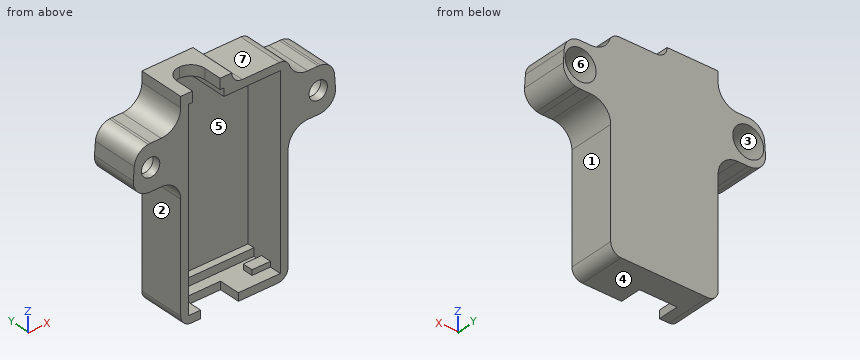
from build123d import *

# Parameters (mm, degrees)
SKETCH1_W           = 20.5
SKETCH1_H           = 38.5
SKETCH1_R           = 4.25
SKETCH1_R_2         = 1.75
BOSS_EXTRUDE1_DEPTH = 1.5
SKETCH2_W           = 20.5
SKETCH2_H           = 38.5
BOSS_EXTRUDE2_DEPTH = 7.35
SKETCH3_W           = 17.5
SKETCH3_H           = 35.5
SKETCH3_W_2         = 6.75
SKETCH3_H_2         = 1.5
CUT_EXTRUDE1_DEPTH  = 7.35
SKETCH4_W           = 7.2
SKETCH4_H           = 1.5
CUT_EXTRUDE2_DEPTH  = 4.05
SKETCH6_W           = 17.5
SKETCH6_H           = 1.5
BOSS_EXTRUDE3_DEPTH = 1.35
SKETCH7_W           = 3.5
SKETCH7_H           = 2
BOSS_EXTRUDE4_DEPTH = 1
SKETCH8_R           = 2.95
BOSS_EXTRUDE5_DEPTH = 7.35
FILLET2_R           = 3.75
CUT_EXTRUDE4_START  = -8.85
CUT_EXTRUDE4_DEPTH  = 8.85
FILLET5_R           = 3
SKETCH10_W          = 9.75
SKETCH10_H          = 2
BOSS_EXTRUDE6_DEPTH = 8.85
CUT_EXTRUDE5_REACH  = 47.729
FILLET4_R           = 2


with BuildPart() as part:
    # Sketch1 → Boss-Extrude1 (new body)
    # profile 1 of 5: a face of its own
    with BuildSketch(Plane(origin=(0, 0, 0), x_dir=(1, 0, 0), z_dir=(0, 1, 0))):
        with Locations((0, 11.25)):
            Rectangle(SKETCH1_W, SKETCH1_H)
    # profile 2 of 5: a face of its own
    with BuildSketch(Plane(origin=(0, 0, 0), x_dir=(1, 0, 0), z_dir=(0, 1, 0))):
        with BuildLine():
            Line((-10.25, -4.25), (-10.25, 4.25))
            Line((-10.25, 4.25), (-16, 4.25))
            ThreePointArc((-16, 4.25), (-12.99479618, 3.00520382), (-11.75, 0))
            ThreePointArc((-11.75, 0), (-12.99479618, -3.00520382), (-16, -4.25))
            Line((-16, -4.25), (-10.25, -4.25))
        make_face()
    # profile 3 of 5: a face of its own
    with BuildSketch(Plane(origin=(0, 0, 0), x_dir=(1, 0, 0), z_dir=(0, 1, 0))):
        with Locations((-16, 0)):
            Circle(SKETCH1_R)
        with Locations(Location((-16, 0, 0), (0, 0, 270))):
            Circle(SKETCH1_R_2, mode=Mode.SUBTRACT)
    # profile 4 of 5: a face of its own
    with BuildSketch(Plane(origin=(0, 0, 0), x_dir=(1, 0, 0), z_dir=(0, 1, 0))):
        with BuildLine():
            Line((16, 4.25), (10.25, 4.25))
            Line((10.25, 4.25), (10.25, -4.25))
            Line((10.25, -4.25), (16, -4.25))
            ThreePointArc((16, -4.25), (11.75, 0), (16, 4.25))
        make_face()
    # profile 5 of 5: a face of its own
    with BuildSketch(Plane(origin=(0, 0, 0), x_dir=(1, 0, 0), z_dir=(0, 1, 0))):
        with Locations((16, 0)):
            Circle(SKETCH1_R)
        with Locations(Location((16, 0, 0), (0, 0, 270))):
            Circle(SKETCH1_R_2, mode=Mode.SUBTRACT)
    extrude(amount=BOSS_EXTRUDE1_DEPTH)

    # Sketch2 → Boss-Extrude2 (add)
    with BuildSketch(Plane(origin=(0, 1.5, 0), x_dir=(1, 0, 0), z_dir=(0, 1, 0))):
        with Locations((0, 11.25)):
            Rectangle(SKETCH2_W, SKETCH2_H)
    extrude(amount=BOSS_EXTRUDE2_DEPTH)

    # Sketch3 → Cut-Extrude1 (cut)
    with BuildSketch(Plane.XZ):
        with Locations((0, -11.25)):
            Rectangle(SKETCH3_W, SKETCH3_H)
        with Locations((-5.375, 7.25)):
            Rectangle(SKETCH3_W_2, SKETCH3_H_2)
    extrude(amount=-CUT_EXTRUDE1_DEPTH, mode=Mode.SUBTRACT)

    # Sketch4 → Cut-Extrude2 (cut)
    with BuildSketch(Plane.XZ):
        with Locations((-2.85, -29.75)):
            Rectangle(SKETCH4_W, SKETCH4_H)
    extrude(amount=-CUT_EXTRUDE2_DEPTH, mode=Mode.SUBTRACT)

    # Sketch6 → Boss-Extrude3 (add)
    with BuildSketch(Plane.XZ.offset(-7.35)):
        with Locations((0, -28.25)):
            Rectangle(SKETCH6_W, SKETCH6_H)
    extrude(amount=BOSS_EXTRUDE3_DEPTH)

    # Sketch7 → Boss-Extrude4 (add)
    with BuildSketch(Plane.XY.offset(-29)):
        with Locations((7, 3.25)):
            Rectangle(SKETCH7_W, SKETCH7_H)
    extrude(amount=BOSS_EXTRUDE4_DEPTH)

    # Sketch8 → Boss-Extrude5 (add)
    # profile 1 of 2: a face of its own
    with BuildSketch(Plane(origin=(0, 1.5, 0), x_dir=(1, 0, 0), z_dir=(0, 1, 0))):
        with BuildLine():
            Line((-10.25, -4.25), (-10.25, 4.25))
            Line((-10.25, 4.25), (-16, 4.25))
            ThreePointArc((-16, 4.25), (-20.25, 0), (-16, -4.25))
            Line((-16, -4.25), (-10.25, -4.25))
        make_face()
        with Locations(Location((-16, 0, 0), (0, 0, 270))):
            Circle(SKETCH8_R, mode=Mode.SUBTRACT)
    # profile 2 of 2: a face of its own
    with BuildSketch(Plane(origin=(0, 1.5, 0), x_dir=(1, 0, 0), z_dir=(0, 1, 0))):
        with BuildLine():
            Line((10.25, 4.25), (10.25, -4.25))
            Line((10.25, -4.25), (16, -4.25))
            ThreePointArc((16, -4.25), (20.25, 0), (16, 4.25))
            Line((16, 4.25), (10.25, 4.25))
        make_face()
        with Locations(Location((16, 0, 0), (0, 0, 270))):
            Circle(SKETCH8_R, mode=Mode.SUBTRACT)
    extrude(amount=BOSS_EXTRUDE5_DEPTH)

    # Fillet2
    fillet2_edges = [part.edges().sort_by_distance(p)[0] for p in [
        (10.25, 4.425, -4.25),
        (10.25, 4.425, 4.25),
        (-10.25, 4.425, 4.25),
        (-10.25, 4.425, -4.25),
    ]]
    fillet(fillet2_edges, radius=FILLET2_R - 0.0001)  # a hair under: the kernel refuses the full size

    # Sketch9 → Cut-Extrude4 (cut)
    with BuildSketch(Plane(origin=(0, 8.85, 0), x_dir=(1, 0, 0), z_dir=(0, 1, 0)).offset(CUT_EXTRUDE4_START)):
        with BuildLine():
            Line((-24.982948352, 53.686308531), (-20.952771504, -3.947905519))
            ThreePointArc((-20.952771504, -3.947905519), (-19.171836931, -8.143524448), (-15.185360396, -10.353264474))
            Line((-15.185360396, -10.353264474), (-1.215537244, -12.816521212))
            ThreePointArc((-1.215537244, -12.816521212), (0, -12.922866941), (1.215537244, -12.816521212))
            Line((1.215537244, -12.816521212), (15.185360396, -10.353264474))
            ThreePointArc((15.185360396, -10.353264474), (19.171836931, -8.143524448), (20.952771504, -3.947905519))
            Line((20.952771504, -3.947905519), (24.982948352, 53.686308531))
            ThreePointArc((24.982948352, 53.686308531), (24.995735789, 53.930307371), (25, 54.174603847))
            Line((25, 54.174603847), (25, 107.825396153))
            ThreePointArc((25, 107.825396153), (24.995735789, 108.069692629), (24.982948352, 108.313691469))
            Line((24.982948352, 108.313691469), (20.952771504, 165.947905519))
            ThreePointArc((20.952771504, 165.947905519), (19.171836931, 170.143524448), (15.185360396, 172.353264474))
            Line((15.185360396, 172.353264474), (1.215537244, 174.816521212))
            ThreePointArc((1.215537244, 174.816521212), (0, 174.922866941), (-1.215537244, 174.816521212))
            Line((-1.215537244, 174.816521212), (-15.185360396, 172.353264474))
            ThreePointArc((-15.185360396, 172.353264474), (-19.171836931, 170.143524448), (-20.952771504, 165.947905519))
            Line((-20.952771504, 165.947905519), (-24.982948352, 108.313691469))
            ThreePointArc((-24.982948352, 108.313691469), (-24.995735789, 108.069692629), (-25, 107.825396153))
            Line((-25, 107.825396153), (-25, 54.174603847))
            ThreePointArc((-25, 54.174603847), (-24.995735789, 53.930307371), (-24.982948352, 53.686308531))
        make_face()
        with BuildLine():
            Line((-18.957643404, 165.808392572), (-22.987820251, 108.174178521))
            ThreePointArc((-22.987820251, 108.174178521), (-22.996954135, 107.999893636), (-23, 107.825396153))
            Line((-23, 107.825396153), (-23, 54.174603847))
            ThreePointArc((-23, 54.174603847), (-22.996954135, 54.000106364), (-22.987820251, 53.825821479))
            Line((-22.987820251, 53.825821479), (-18.957643404, -3.808392572))
            ThreePointArc((-18.957643404, -3.808392572), (-17.68554728, -6.805263235), (-14.838064041, -8.383648968))
            Line((-14.838064041, -8.383648968), (-0.868240888, -10.846905706))
            ThreePointArc((-0.868240888, -10.846905706), (0, -10.922866941), (0.868240888, -10.846905706))
            Line((0.868240888, -10.846905706), (14.838064041, -8.383648968))
            ThreePointArc((14.838064041, -8.383648968), (17.68554728, -6.805263235), (18.957643404, -3.808392572))
            Line((18.957643404, -3.808392572), (22.987820251, 53.825821479))
            ThreePointArc((22.987820251, 53.825821479), (22.996954135, 54.000106364), (23, 54.174603847))
            Line((23, 54.174603847), (23, 107.825396153))
            ThreePointArc((23, 107.825396153), (22.996954135, 107.999893636), (22.987820251, 108.174178521))
            Line((22.987820251, 108.174178521), (18.957643404, 165.808392572))
            ThreePointArc((18.957643404, 165.808392572), (17.68554728, 168.805263235), (14.838064041, 170.383648968))
            Line((14.838064041, 170.383648968), (0.868240888, 172.846905706))
            ThreePointArc((0.868240888, 172.846905706), (0, 172.922866941), (-0.868240888, 172.846905706))
            Line((-0.868240888, 172.846905706), (-14.838064041, 170.383648968))
            ThreePointArc((-14.838064041, 170.383648968), (-17.68554728, 168.805263235), (-18.957643404, 165.808392572))
        make_face(mode=Mode.SUBTRACT)
    extrude(amount=CUT_EXTRUDE4_DEPTH, mode=Mode.SUBTRACT)

    # Fillet5
    fillet5_edges = [part.edges().sort_by_distance(p)[0] for p in [
        (-19.402072162, 4.425, -2.547234776),
        (-19.014456867, 4.425, 2.995922195),
        (19.014456867, 4.425, 2.995922195),
        (19.402072162, 4.425, -2.547234776),
    ]]
    fillet(fillet5_edges, radius=FILLET5_R)

    # Sketch10 → Boss-Extrude6 (add)
    with BuildSketch(Plane(origin=(0, 0, 0), x_dir=(1, 0, 0), z_dir=(0, 1, 0))):
        with Locations((-5.375, -9)):
            Rectangle(SKETCH10_W, SKETCH10_H)
    extrude(amount=BOSS_EXTRUDE6_DEPTH)

    # Sketch11 → Cut-Extrude5 (cut, up to next)
    with BuildSketch(Plane.XY.offset(10), mode=Mode.PRIVATE) as cut_extrude5_sk1:
        with BuildLine():
            ThreePointArc((-2.725, 3.5), (-3.50116703, 5.37383297), (-5.375, 6.15))
            Line((-5.375, 6.15), (-5.375, 0.85))
            ThreePointArc((-5.375, 0.85), (-3.50116703, 1.62616703), (-2.725, 3.5))
        make_face()
    cut_extrude5_tool1 = extrude(cut_extrude5_sk1.sketch, amount=-CUT_EXTRUDE5_REACH, mode=Mode.PRIVATE) & part.part
    # Sketch11 → Cut-Extrude5 (cut, up to next)
    with BuildSketch(Plane.XY.offset(10), mode=Mode.PRIVATE) as cut_extrude5_sk2:
        with BuildLine():
            Line((-5.375, 0.85), (-5.375, 6.15))
            ThreePointArc((-5.375, 6.15), (-7.24883297, 5.37383297), (-8.025, 3.5))
            ThreePointArc((-8.025, 3.5), (-7.24883297, 1.62616703), (-5.375, 0.85))
        make_face()
    cut_extrude5_tool2 = extrude(cut_extrude5_sk2.sketch, amount=-CUT_EXTRUDE5_REACH, mode=Mode.PRIVATE) & part.part
    # Sketch11 → Cut-Extrude5 (cut, up to next)
    with BuildSketch(Plane.XY.offset(10), mode=Mode.PRIVATE) as cut_extrude5_sk3:
        with BuildLine():
            ThreePointArc((-2.725, 3.5), (-3.50116703, 5.37383297), (-5.375, 6.15))
            Line((-5.375, 6.15), (-5.375, 0.85))
            ThreePointArc((-5.375, 0.85), (-3.50116703, 1.62616703), (-2.725, 3.5))
        make_face()
    cut_extrude5_tool3 = extrude(cut_extrude5_sk3.sketch, amount=-CUT_EXTRUDE5_REACH, mode=Mode.PRIVATE) & part.part
    # Sketch11 → Cut-Extrude5 (cut, up to next)
    with BuildSketch(Plane.XY.offset(10), mode=Mode.PRIVATE) as cut_extrude5_sk4:
        with BuildLine():
            Line((-5.375, 0.85), (-5.375, 6.15))
            ThreePointArc((-5.375, 6.15), (-7.24883297, 5.37383297), (-8.025, 3.5))
            ThreePointArc((-8.025, 3.5), (-7.24883297, 1.62616703), (-5.375, 0.85))
        make_face()
    cut_extrude5_tool4 = extrude(cut_extrude5_sk4.sketch, amount=-CUT_EXTRUDE5_REACH, mode=Mode.PRIVATE) & part.part
    # Sketch11 → Cut-Extrude5 (cut, up to next)
    with BuildSketch(Plane.XY.offset(10), mode=Mode.PRIVATE) as cut_extrude5_sk5:
        with BuildLine():
            Line((-5.375, 0), (-5.375, 0.85))
            ThreePointArc((-5.375, 0.85), (-7.24883297, 1.62616703), (-8.025, 3.5))
            Line((-8.025, 3.5), (-8.025, 0))
            Line((-8.025, 0), (-5.375, 0))
        make_face()
    cut_extrude5_tool5 = extrude(cut_extrude5_sk5.sketch, amount=-CUT_EXTRUDE5_REACH, mode=Mode.PRIVATE) & part.part
    # Sketch11 → Cut-Extrude5 (cut, up to next)
    with BuildSketch(Plane.XY.offset(10), mode=Mode.PRIVATE) as cut_extrude5_sk6:
        with BuildLine():
            ThreePointArc((-2.725, 3.5), (-3.50116703, 1.62616703), (-5.375, 0.85))
            Line((-5.375, 0.85), (-5.375, 0))
            Line((-5.375, 0), (-2.725, 0))
            Line((-2.725, 0), (-2.725, 3.5))
        make_face()
    cut_extrude5_tool6 = extrude(cut_extrude5_sk6.sketch, amount=-CUT_EXTRUDE5_REACH, mode=Mode.PRIVATE) & part.part
    add(cut_extrude5_tool1.solids().sort_by_distance((-4.250305, 3.5, 10))[0], mode=Mode.SUBTRACT)
    add(cut_extrude5_tool2.solids().sort_by_distance((-6.499695, 3.5, 10))[0], mode=Mode.SUBTRACT)
    add(cut_extrude5_tool3.solids().sort_by_distance((-4.250305, 3.5, 10))[0], mode=Mode.SUBTRACT)
    add(cut_extrude5_tool4.solids().sort_by_distance((-6.499695, 3.5, 10))[0], mode=Mode.SUBTRACT)
    add(cut_extrude5_tool5.solids().sort_by_distance((-6.993859, 0.832642, 10))[0], mode=Mode.SUBTRACT)
    add(cut_extrude5_tool6.solids().sort_by_distance((-3.756141, 0.832642, 10))[0], mode=Mode.SUBTRACT)

    # Fillet4
    fillet4_edges = [part.edges().sort_by_distance(p)[0] for p in [
        (10.25, 4.425, 8),
        (10.25, 4.425, -30.5),
        (-10.25, 4.425, -30.5),
        (-0.5, 4.425, 8),
    ]]
    fillet(fillet4_edges, radius=FILLET4_R - 0.0001)  # a hair under: the kernel refuses the full size


solid = part.part
Design review of the part built by this model. Coordinates are the model's own, in mm. Face numbers are marked on the shaded views. A direction names the side the tool comes from. Give positions to 0.01 mm unless a question says otherwise; leave off trailing zeros. Loops run counter-clockwise (first coordinate to the right, second up) from the corner with the lowest first, then second, coordinate; pieces in that order, holes last. Notation, with made-up numbers: M -23,79 L 15,79 A15 ccw 15,87 Z; hole C -3,27 d6. An arc over 180 degrees is marked long. Write item = value, one per line.
Q1. For the marked faces 1, 2 and 3, list the 3-axis set-ups (+Z, -Z, +X, -X, +Y, -Y) from which the entire face can be reached by the end or side of a thin tool; tool diameter is ignored.
Output values:
face_1 = -Z, +X, +Y, -Y
face_2 = -Z, -X, +Y, -Y
face_3 = +Y
Q2. To check wall thickness, follow line 1 (X direction, y = 2.5, z = -8); line 2 (X direction, y = 3.5, z = -1); line 3 (Z direction, x = 2.5, y = 3.5). State the ranges of each line that lie inside material, in increasing order. Write a range as [from, to].
Output values:
line_1 = [-10.25, -8.75], [8.75, 10.25]
line_2 = [-19.29, -18.78], [-13.22, -8.75], [8.75, 13.22], [18.78, 19.29]
line_3 = [-30.5, -29], [6.5, 8]
Q3. We need section A-A (z = -21). Give the boundary of the cut face in (x, y), plus the area to 3 significant figures.
Output values:
outline = M -10.25,0 L -8.75,0 L -8.75,7.35 L 8.75,7.35 L 8.75,0 L 10.25,0 L 10.25,8.85 L -10.25,8.85 Z
area = 52.8 mm^2
Q4. We need section D-D (x = -11). Give the boundary of the cut face in (y, z).
Output values:
outline = M 0,-5.75 L 8.85,-5.75 L 8.85,5.75 L 0,5.75 Z
Q5. We need section C-C (z = 0). Give the boundary of the cut face in (x, y), plus the area to 3 significant figures.
Output values:
outline = M -19.22,0 L -17.75,0 L -17.75,1.5 L -18.95,1.5 L -18.95,8.85 L -19.22,8.85 Z; M -14.25,0 L -8.75,0 L -8.75,7.35 L 8.75,7.35 L 8.75,0 L 14.25,0 L 14.25,1.5 L 13.05,1.5 L 13.05,8.85 L -13.05,8.85 L -13.05,1.5 L -14.25,1.5 Z; M 17.75,0 L 19.22,0 L 19.22,8.85 L 18.95,8.85 L 18.95,1.5 L 17.75,1.5 Z
area = 114 mm^2
Q6. Draft analysis for pull direction Z (two halves, no side actions). For the marked faces 4, 5, 6 and 7, state which applies: +Z half, -Z half, draft (parallel to the pull), parting line (faces both ways), or undercut.
Output values:
face_4 = -Z half
face_5 = undercut
face_6 = undercut
face_7 = +Z half
Q7. We need section B-B (y = 2.75). Count the separate pieces of the cut face and the enclosed holes in it, plus the area to 3 significant figures.
Output values:
separate_pieces = 2
enclosed_holes = 2
area = 260 mm^2
Q8. Insertion check: pin 1 (3.5 mm diameter, centred on y = 3.5, z = -9, fed in from +X); pin 2 (5 mm diameter, centred on y = 1.5, z = -4.5, fed in from +X); pin 3 (2 mm diameter, centred on x = 15.5, y = 3.5, fed in from -Z). Each pin has a flat end and moves straight along its axis. Give the tip position at first contact, or say it passes through.
Output values:
pin_1 = 10.33
pin_2 = 19.2
pin_3 = -4.25
